Can you work these out from the model? Positions are in its coordinate system, mm. A direction names the side the tool comes from. Round coordinates to 2 decimals unless told otherwise and drop trailing zeros. Order: outer loops, then holes, each group sorted by start corner. A loop starts at its lowest first (then second) coordinate and runs counter-clockwise, first axis right, second up. Notation, with made-up numbers: M 78,55 L 133,55 A37 ccw 133,91 Z; hole C -28,77 d10. An arc over 180 degrees is marked long. Answer as a JSON object with one key per item and string values. Group by question number.
from build123d import *

# Parameters (mm, degrees)
F0_W     = 25.4
F0_H     = 25.4
F1_DEPTH = 25.4
F2_W     = 5.08
F2_H     = 20.32
F3_DEPTH = 25.4
F5_DEPTH = 25.4
F7_DEPTH = 25.4


with BuildPart() as f1:
    # F0 (on Top) → F1 (new body)
    with BuildSketch(Plane.XY):
        Rectangle(F0_W, F0_H)
    extrude(amount=F1_DEPTH)

    # F2 (on face) → F3 (cut)
    with BuildSketch(Plane.XY.offset(25.4)):
        with Locations((-5.08, 2.54)):
            Rectangle(F2_W, F2_H)
        with Locations((5.08, 2.54)):
            Rectangle(F2_W, F2_H)
    extrude(amount=-F3_DEPTH, mode=Mode.SUBTRACT)

    # F4 (on face) → F5 (cut)
    with BuildSketch(Plane.YZ.offset(12.7)):
        with BuildLine():
            Line((5.08, 20.32), (-7.62, 20.32))
            Line((-7.62, 20.32), (-7.62, 15.24))
            Line((-7.62, 15.24), (5.08, 15.24))
            ThreePointArc((5.08, 15.24), (7.62, 17.78), (5.08, 20.32))
        make_face()
        with BuildLine():
            Line((5.08, 10.16), (-7.62, 10.16))
            Line((-7.62, 10.16), (-7.62, 5.08))
            Line((-7.62, 5.08), (5.08, 5.08))
            ThreePointArc((5.08, 5.08), (7.62, 7.62), (5.08, 10.16))
        make_face()
        with BuildLine():
            ThreePointArc((5.08, 25.4), (10.4681536726, 23.1681536726), (12.7, 17.78))
            Line((12.7, 17.78), (12.7, 25.4))
            Line((12.7, 25.4), (5.08, 25.4))
        make_face()
        with BuildLine():
            ThreePointArc((10.7596126628, 12.7), (12.1983933753, 10.3389843241), (12.7, 7.62))
            Line((12.7, 7.62), (12.7, 17.78))
            ThreePointArc((12.7, 17.78), (12.1983933753, 15.0610156759), (10.7596126628, 12.7))
        make_face()
        with BuildLine():
            ThreePointArc((12.7, 7.62), (10.4681536726, 2.2318463274), (5.08, 0))
            Line((5.08, 0), (12.7, 0))
            Line((12.7, 0), (12.7, 7.62))
        make_face()
    extrude(amount=-F5_DEPTH, mode=Mode.SUBTRACT)

    # F6 (on face) → F7 (cut)
    with BuildSketch(Plane.XZ.offset(12.7)):
        Polygon((12.7, 15.24), (12.7, 20.32), (-7.62, 20.32), (-7.62, 15.24), (-7.62, 5.08), (-2.54, 5.08), (7.62, 5.08), (7.62, 10.16), (-2.54, 10.16), (-2.54, 15.24), align=None)
    extrude(amount=-F7_DEPTH, mode=Mode.SUBTRACT)


solid = f1.part
Item 1: I need wall thicknesses on line 1 (Z direction, x = 10.75, y = -7); line 2 (X direction, y = 2, z = 10.25); line 3 (X direction, y = -11.25, z = 14). Which ranges of each line are inside material? Lowest first, please.
Item 2: Suppose I cut it at D-D, the plane y = 1. State how many separate pieces and enclosed holes the cut face has, and give its area (3 significant figures).
Item 3: On a 3-axis mill with a long thin cutter (end or side, diameter ignored), from which of +Z, -Z, +X, -X, +Y, -Y can I reach the whole of each face in a straight line? I mean faces 5 (the face through (0, -3, 20.32)), 6 (the face through (10.196, 11.647, 13.914)), 7 (the face through (2.54, 2, 3)). Say none if no direction works.
Item 4: I'm going to push flat-ended pins straight in: pin 1 Ø1 at (x, z) = (9.5, 4.5) entering from +Y; pin 2 Ø8 at (x, z) = (-1.5, 20.5) entering from +Y; pin 3 Ø1.5 at (x, z) = (8.5, 19.5) entering from -Y; pin 4 Ø2.5 at (x, z) = (6.5, 22) entering from +Y. Where does each tip first touch, or does it pass through?
Item 5: If we mould it in two halves opening along Y, with no side actions, what happens to faces 1 (the face through (7.62, -10, 8)), 2 (the face through (-10.12, 7.62, 7.56)), 3 (the face through (-10, -1, 20.32)), 4 (the face through (5, -7.62, 3))? For each: +Y half, -Y half, draft (parallel to the pull), parting line (faces both ways), or undercut.
Item 6: Suppose I cut it at A-A, the plane x = 5.25. Write out the boundary of the cut face in (y, z), and give its area (3 significant figures).
Item 7: Suppose I cut it at C-C, the plane z = 8. Write out the boundary of the cut face in (x, y).
Item 8: Suppose I cut it at B-B, the plane y = 9.5. Write out the boundary of the cut face in (x, z), and give its area (3 significant figures).
Computed:
{
 "1": {"line 1": "z = 0 to 5.08, 10.16 to 15.24, 20.32 to 25.4", "line 2": "x = -12.7 to -7.62, -2.54 to 2.54, 7.62 to 12.7", "line 3": "x = -12.7 to -7.62, -2.54 to 12.7"},
 "2": {"separate pieces": "9", "enclosed holes": "0", "area": "232 mm^2"},
 "3": {"face 5": "+X, +Y, -Y", "face 6": "+X, -X, +Y", "face 7": "+Z, -Z, +Y"},
 "4": {"pin 1": "stops at y = 12.24", "pin 2": "stops at y = 12.26", "pin 3": "passes through", "pin 4": "stops at y = 11.76"},
 "5": {"face 1": "draft", "face 2": "undercut", "face 3": "undercut", "face 4": "+Y half"},
 "6": {"outline": "M -12.7,0 L -7.62,0 L -7.62,5.08 L -12.7,5.08 Z; M -12.7,10.16 L -7.62,10.16 L -7.62,15.24 L -12.7,15.24 Z; M -12.7,20.32 L -7.62,20.32 L -7.62,25.4 L -12.7,25.4 Z", "area": "77.4 mm^2"},
 "7": {"outline": "M -12.7,-12.7 L -7.62,-12.7 L -7.62,-7.62 L -12.7,-7.62 Z; M -12.7,7.59 L -7.62,7.59 L -7.62,12.69 L -12.7,12.69 Z; M 7.62,-12.7 L 12.7,-12.7 L 12.7,-7.62 L 7.62,-7.62 Z; M 7.62,7.59 L 12.7,7.59 L 12.7,12.69 L 7.62,12.69 Z"},
 "8": {"outline": "M -12.7,1.41 L -7.62,1.41 L -7.62,23.99 L -12.7,23.99 Z; M -2.54,1.41 L 2.54,1.41 L 2.54,5.08 L -2.54,5.08 Z; M -2.54,10.16 L 2.54,10.16 L 2.54,15.24 L -2.54,15.24 Z; M -2.54,20.32 L 2.54,20.32 L 2.54,23.99 L -2.54,23.99 Z; M 7.62,1.41 L 12.7,1.41 L 12.7,15.24 L 7.62,15.24 Z; M 7.62,20.32 L 12.7,20.32 L 12.7,23.99 L 7.62,23.99 Z", "area": "267 mm^2"}
}
